```python
from build123d import *

# Parameters (mm, degrees)
BOSS_EXTRUDE1_DEPTH       = 40
M3X0_5_TAPPED_HOLE1_D     = 2.5
M3X0_5_TAPPED_HOLE1_DEPTH = 6
M3X0_5_TAPPED_HOLE1_TIP   = 0.751075774


with BuildPart() as part:
    # Sketch2 → Boss-Extrude1 (new body)
    with BuildSketch(Plane.XY):
        Polygon((0, 0), (0, 8), (20, 8), (20, 0), (14.5, 0), (14.5, 4.5), (5.5, 4.5), (5.5, 0), align=None)
    extrude(amount=BOSS_EXTRUDE1_DEPTH)

    # M3x0.5 Tapped Hole1
    with Locations(Plane(origin=(0, 8, 0), x_dir=(1, 0, 0), z_dir=(0, 1, 0))):
        with Locations((2.5, -28), (2.5, -12), (17.5, -28), (17.5, -12)):
            Hole(M3X0_5_TAPPED_HOLE1_D / 2, depth=M3X0_5_TAPPED_HOLE1_DEPTH)
            with Locations((0, 0, -(M3X0_5_TAPPED_HOLE1_DEPTH + M3X0_5_TAPPED_HOLE1_TIP / 2))):  # 118° drill point
                Cone(0, M3X0_5_TAPPED_HOLE1_D / 2, M3X0_5_TAPPED_HOLE1_TIP, mode=Mode.SUBTRACT)


solid = part.part
```
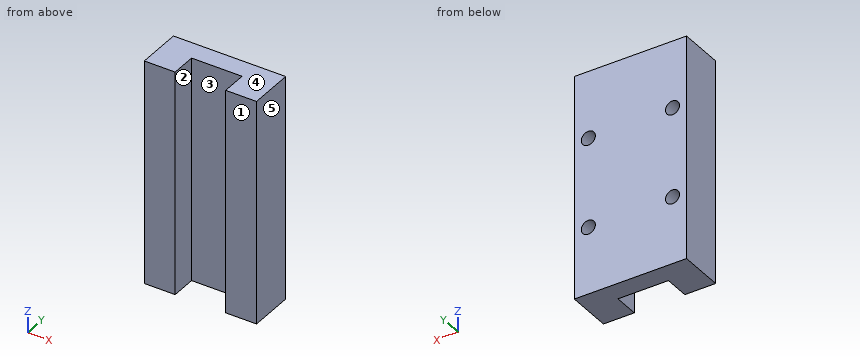
Here's how the part is built. I have some questions about the finished solid (model axes, mm). Face numbers are marked on the shaded views. A direction names the side the tool comes from. Give positions to 0.01 mm unless a question says otherwise; leave off trailing zeros. Order: outer loops, then holes, each group sorted by start corner. A loop starts at its lowest first (then second) coordinate and runs counter-clockwise, first axis right, second up. Notation, with made-up numbers: (66.25, -35) - (84.25, -35) arc R22 ccw to (84.25, 2) - close; hole circle Ø9 at (25.25, 87). An arc over 180 degrees is marked (long way). Answer as a JSON object with one key per item and string values. Group by question number.
Item 1: If we mould it in two halves opening along X, with no side actions, what happens to the marked faces 3, 4 and 5? For each: pulls with the +X half, pulls with the -X half, needs draft (parallel to the pull), parting line crosses it, or undercut.
Item 2: If we section it at D-D on y = 6: Please give me the cut outline in (x, z).
Item 3: For P1, Ø10, axis at x = 8, z = 14.5, coming from the -Y side, with a flat end and sliding along its axis, tell me the tip position at first contact or that it passes through.
Item 4: If we section it at B-B on y = 0.5: Please give me the cut outline in (x, z).
Item 5: Please list where these lines run through material, in increasing order: probe 1 along Z at (x, y) = (17.5, 3.25); probe 2 along X at (y, z) = (5.7, 12); probe 3 along X at (y, z) = (4.35, 28).
Item 6: Which directions (+Z, -Z, +X, -X, +Y, -Y) give clear straight access to the entire face, cutting with the end or side of a thin tool? Please do the marked faces 1 and 2.
Item 7: If we section it at A-A on y = 2.5: Please give me the cut outline in (x, z).
Item 8: If we section it at C-C on z = 15: Please give me the cut outline in (x, y).
Result set:
{
 "1": {"face 3": "undercut", "face 4": "needs draft", "face 5": "pulls with the +X half"},
 "2": {"outline": "(0, 0) - (20, 0) - (20, 40) - (0, 40) - close; hole circle Ø2.5 at (2.5, 12); hole circle Ø2.5 at (2.5, 28); hole circle Ø2.5 at (17.5, 12); hole circle Ø2.5 at (17.5, 28)"},
 "3": {"P1": "y = 0"},
 "4": {"outline": "(0, 0) - (5.5, 0) - (5.5, 40) - (0, 40) - close; (14.5, 0) - (20, 0) - (20, 40) - (14.5, 40) - close"},
 "5": {"probe 1": "0 to 10.75, 13.25 to 26.75, 29.25 to 40", "probe 2": "0 to 1.25, 3.75 to 16.25, 18.75 to 20", "probe 3": "0 to 1.25, 3.75 to 5.5, 14.5 to 16.25, 18.75 to 20"},
 "6": {"face 1": "+Z, -Z, +X, -X, -Y", "face 2": "+Z, -Z, -Y"},
 "7": {"outline": "(0, 0) - (5.5, 0) - (5.5, 40) - (0, 40) - close; (14.5, 0) - (20, 0) - (20, 40) - (14.5, 40) - close; hole circle Ø2.5 at (2.5, 12); hole circle Ø2.5 at (2.5, 28); hole circle Ø2.5 at (17.5, 12); hole circle Ø2.5 at (17.5, 28)"},
 "8": {"outline": "(0, 0) - (5.5, 0) - (5.5, 4.5) - (14.5, 4.5) - (14.5, 0) - (20, 0) - (20, 8) - (0, 8) - close"}
}
